Part model, mm, in its own coordinate system. A direction names the side the tool comes from. Round coordinates to 2 decimals unless told otherwise and drop trailing zeros. Order: outer loops, then holes, each group sorted by start corner. A loop starts at its lowest first (then second) coordinate and runs counter-clockwise, first axis right, second up. Notation, with made-up numbers: (71, 41.5) -> (104, 41.5) arc R30 cw to (104, 70.5) -> close; hole circle Ø2 at (26, 57.25). An arc over 180 degrees is marked (long way). Use CSV: the item, a comma, the result in double quotes.
```python
from build123d import *

# Parameters (mm, degrees)
SKETCH2_W           = 305
SKETCH2_H           = 150
BOSS_EXTRUDE1_DEPTH = 5
SKETCH3_W           = 13
SKETCH3_H           = 6.5
CUT_EXTRUDE1_DEPTH  = 305
SKETCH4_W           = 160
SKETCH4_H           = 110
CUT_EXTRUDE2_DEPTH  = 3
FILLET1_R           = 5
SKETCH5_W           = 135
SKETCH5_H           = 80
CUT_EXTRUDE3_DEPTH  = 8


with BuildPart() as part:
    # Sketch2 → Boss-Extrude1 (new body, symmetric)
    with BuildSketch(Plane(origin=(0, 0, 0), x_dir=(1, 0, 0), z_dir=(0, 1, 0))):
        Rectangle(SKETCH2_W, SKETCH2_H)
    extrude(amount=BOSS_EXTRUDE1_DEPTH, both=True)

    # Sketch3 → Cut-Extrude1 (cut)
    with BuildSketch(Plane(origin=(152.5, 0, 0), x_dir=(0, 0, -1), z_dir=(1, 0, 0))):
        with Locations((-68.5, -1.75)):
            Rectangle(SKETCH3_W, SKETCH3_H)
        with Locations((68.5, -1.75)):
            Rectangle(SKETCH3_W, SKETCH3_H)
    extrude(amount=-CUT_EXTRUDE1_DEPTH, mode=Mode.SUBTRACT)

    # Sketch4 → Cut-Extrude2 (cut)
    with BuildSketch(Plane(origin=(0, 5, 0), x_dir=(1, 0, 0), z_dir=(0, 1, 0))):
        with Locations((2.5, 0)):
            Rectangle(SKETCH4_W, SKETCH4_H)
    extrude(amount=-CUT_EXTRUDE2_DEPTH, mode=Mode.SUBTRACT)

    # Fillet1
    fillet1_edges = [part.edges().sort_by_distance(p)[0] for p in [
        (-77.5, 3.5, 55),
        (-77.5, 3.5, -55),
        (82.5, 3.5, -55),
        (82.5, 3.5, 55),
    ]]
    fillet(fillet1_edges, radius=FILLET1_R)

    # Sketch5 → Cut-Extrude3 (cut, through all)
    with BuildSketch(Plane(origin=(0, 2, 0), x_dir=(1, 0, 0), z_dir=(0, 1, 0))):
        Rectangle(SKETCH5_W, SKETCH5_H)
    extrude(amount=-CUT_EXTRUDE3_DEPTH, mode=Mode.SUBTRACT)


solid = part.part
```
(1) Which spindle directions (+Z, -Z, +X, -X, +Y, -Y) get a long thin tool onto all of the face, cutting with end or side? Do faces 1 (the face through (-2, 5, -68)), 2 (the face through (-1, -1, -40)), 3 (the face through (2, 1.5, 69)), 4 (the face through (1, 2, 48)), 5 (the face through (2, 1.5, -68)). Say none if no direction does.
Reply:
face 1,"+Z, -Z, +X, -X, +Y"
face 2,"+Y, -Y"
face 3,"+Z, +X, -X, -Y"
face 4,"+Y"
face 5,"-Z, +X, -X, -Y"
(2) Drop flat-ended pins along their axis: P1, Ø12, axis at x = 25.5, z = -48.5, coming from the +Y side; P2, Ø1, axis at x = 110, y = -2, coming from the -Z side; P3, Ø10.5, axis at x = 11, z = -70.5, coming from the -Y side. Give the stop position or say it passes through.
Reply:
P1,"y = 2"
P2,"z = -62"
P3,"y = 1.5"
(3) Probe probe 1 along Z at (x, y) = (-65, -2.5); probe 2 along Z at (x, y) = (-14.5, 3); probe 3 along X at (y, z) = (-2.25, 24). List the from-to ranges inside material, lowest first. Write a range as [from, to].
Reply:
probe 1,"[-62, -40], [40, 62]"
probe 2,"[-75, -55], [55, 75]"
probe 3,"[-152.5, -67.5], [67.5, 152.5]"
(4) Cut at A-A, the plane x = 25. Give the cut face in (y, z), then the cut area to 3 significant figures.
Reply:
outline,"(-5, -62) -> (1.5, -62) -> (1.5, -75) -> (5, -75) -> (5, -55) -> (2, -55) -> (2, -40) -> (-5, -40) -> close; (-5, 40) -> (2, 40) -> (2, 55) -> (5, 55) -> (5, 75) -> (1.5, 75) -> (1.5, 62) -> (-5, 62) -> close"
area,"441 mm2"
(5) Cut at C-C, the plane y = -1. Give the cut face in (x, z).
Reply:
outline,"(-152.5, -62) -> (152.5, -62) -> (152.5, 62) -> (-152.5, 62) -> close; hole (-67.5, -40) -> (67.5, -40) -> (67.5, 40) -> (-67.5, 40) -> close"
(6) Cut at D-D, the plane x = 111. Give the cut face in (y, z).
Reply:
outline,"(-5, -62) -> (1.5, -62) -> (1.5, -75) -> (5, -75) -> (5, 75) -> (1.5, 75) -> (1.5, 62) -> (-5, 62) -> close"
(7) Cut at B-B, the plane z = -15.5. Give the cut face in (x, y), then the cut area to 4 significant figures.
Reply:
outline,"(-152.5, -5) -> (-67.5, -5) -> (-67.5, 2) -> (-77.5, 2) -> (-77.5, 5) -> (-152.5, 5) -> close; (67.5, -5) -> (152.5, -5) -> (152.5, 5) -> (82.5, 5) -> (82.5, 2) -> (67.5, 2) -> close"
area,"1,625 mm2"
(8) Pull direction Z, two halves, no side cores. Call faces 6 (the face through (-2, -5, -42)), 7 (the face through (-1, -1, 40)), 8 (the face through (2, -2, -62)): released by +Z, released by -Z, zero draft, split by the parting line, or undercut.
Reply:
face 6,"zero draft"
face 7,"undercut"
face 8,"released by -Z"
